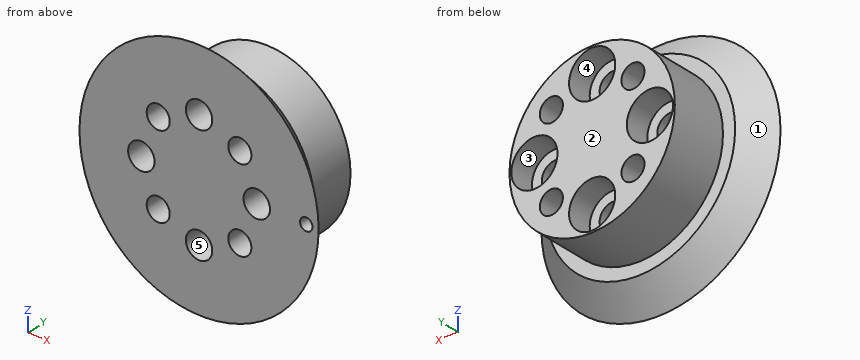
from build123d import *

# Parameters (mm, degrees)
SKETCH2_R                               = 1.4
CUT_EXTRUDE1_DEPTH                      = 23.814469093
CBORE_FOR_M5_HEX_HEAD_BOLT1_D           = 3.2
CBORE_FOR_M5_HEX_HEAD_BOLT1_CBORE_D     = 5.6
CBORE_FOR_M5_HEX_HEAD_BOLT1_CBORE_DEPTH = 3
SKETCH4_R                               = 0.75
CUT_EXTRUDE3_DEPTH                      = 23.814469093


with BuildPart() as part:
    # Sketch1 → Revolve1 (revolve)
    with BuildSketch(Plane.XY, mode=Mode.PRIVATE) as revolve1_sk:
        Polygon((14.5, 0), (11.5, 3), (10.025, 3), (10.025, 10), (0, 10), (0, 0), align=None)
    revolve(revolve1_sk.sketch.rotate(Axis((0, 10, 0), (0, -1, 0)), 180), axis=Axis((0, 10, 0), (0, -1, 0)))

    # Sketch2 → Cut-Extrude1 (cut, through all)
    with BuildSketch(Plane(origin=(0, 10, 0), x_dir=(1, 0, 0), z_dir=(0, 1, 0))):
        with Locations(Location((0, 7, 0), (0, 0, 180))):
            Circle(SKETCH2_R)
        with Locations(Location((4.949747468, 4.949747468, 0), (0, 0, 180))):
            Circle(SKETCH2_R)
        with Locations(Location((7, 0, 0), (0, 0, 180))):
            Circle(SKETCH2_R)
        with Locations(Location((4.949747468, -4.949747468, 0), (0, 0, 180))):
            Circle(SKETCH2_R)
        with Locations(Location((0, -7, 0), (0, 0, 180))):
            Circle(SKETCH2_R)
        with Locations(Location((-4.949747468, -4.949747468, 0), (0, 0, 180))):
            Circle(SKETCH2_R)
        with Locations(Location((-7, 0, 0), (0, 0, 180))):
            Circle(SKETCH2_R)
        with Locations(Location((-4.949747468, 4.949747468, 0), (0, 0, 180))):
            Circle(SKETCH2_R)
    extrude(amount=-CUT_EXTRUDE1_DEPTH, mode=Mode.SUBTRACT)

    # CBORE for M5 Hex Head Bolt1 (through all)
    with Locations(Plane(origin=(0, 10, -7), x_dir=(1, 0, 0), z_dir=(0, 1, 0))):
        with Locations((0, 0), (-7, -7), (0, -14), (7, -7)):
            CounterBoreHole(CBORE_FOR_M5_HEX_HEAD_BOLT1_D / 2, CBORE_FOR_M5_HEX_HEAD_BOLT1_CBORE_D / 2, CBORE_FOR_M5_HEX_HEAD_BOLT1_CBORE_DEPTH)

    # Sketch4 → Cut-Extrude3 (cut, through all)
    with BuildSketch(Plane(origin=(0, 0, 0), x_dir=(1, 0, 0), z_dir=(0, 1, 0))):
        with Locations(Location((13, 0, 0), (0, 0, 90.394644161))):
            Circle(SKETCH4_R)
    extrude(amount=CUT_EXTRUDE3_DEPTH, mode=Mode.SUBTRACT)


solid = part.part
Can you work these out from the model? Positions are in its coordinate system, mm. Face numbers are marked on the shaded views. A direction names the side the tool comes from. Coordinates: 2 decimals unless noted, no trailing zeros. Order: outer loops, then holes, each group sorted by start corner. A loop starts at its lowest first (then second) coordinate and runs counter-clockwise, first axis right, second up. Notation, with made-up numbers: (38, 29.25) - (71, 29.25) arc R25 cw to (71, 66.25) - close; hole circle Ø3 at (75.25, 88.5). An arc over 180 degrees is marked (long way). Answer as a JSON object with one key per item and string values. Group by question number.
Q1. Will these pins go through, and if not, where does the flat tip stop? P1, Ø2, axis at x = 4.95, z = 4.95, coming from the -Y side; P2, Ø6, axis at x = -11, y = 8.5, coming from the -Z side; P3, Ø5, axis at x = 0, z = -7, coming from the +Y side; P4, Ø1, axis at x = 9, y = 2.5, coming from the -Z side.
Q2. We'd pull the mould along Z, two halves only. Please class the marked faces 1, 2 and 3: +Z half, -Z half, draft (parallel to the pull), parting line (faces both ways), or undercut.
Q3. Imagine slicing it at A-A (z = 0). Please give me the cut outline in (x, y) (3 decimals), and give its area (3 significant figures).
Q4. I need wall thicknesses on line 1 (Z direction, x = 0, y = 9.05) (3 decimals); line 2 (X direction, y = 2.75, z = 0.25); line 3 (Z direction, x = -4, y = 1). Which ranges of each line are inside material? Lowest first, please. Write a range as from..to.
Q5. Imagine slicing it at B-B (x = 0). Please give me the cut outline in (y, z) (3 decimals), and give its area (3 significant figures).
Q6. On a 3-axis mill with a long thin cutter (end or side, diameter ignored), from which of +Z, -Z, +X, -X, +Y, -Y can I reach the whole of each face in a straight line? I mean the marked faces 4 and 5. Say none if no direction works.
Determined:
{
 "1": {"P1": "passes through", "P2": "stops at z = -6.04", "P3": "stops at y = 7", "P4": "stops at z = -8.84"},
 "2": {"face 1": "parting line", "face 2": "draft", "face 3": "undercut"},
 "3": {"outline": "(-14.5, 0) - (-8.6, 0) - (-8.6, 7) - (-9.8, 7) - (-9.8, 10) - (-10.025, 10) - (-10.025, 3) - (-11.5, 3) - close; (-5.4, 0) - (5.4, 0) - (5.4, 7) - (4.2, 7) - (4.2, 10) - (-4.2, 10) - (-4.2, 7) - (-5.4, 7) - close; (8.6, 0) - (12.25, 0) - (12.25, 2.25) - (11.5, 3) - (10.025, 3) - (10.025, 10) - (9.8, 10) - (9.8, 7) - (8.6, 7) - close; (13.75, 0) - (14.5, 0) - (13.75, 0.75) - close", "area": "138 mm2"},
 "4": {"line 1": "z = -10.025..-9.8, -4.2..4.2, 9.8..10.025", "line 2": "x = -11.75..-8.58, -5.42..5.42, 8.58..11.75", "line 3": "z = -12.89..-5.98, -3.92..3.92, 5.98..12.89"},
 "5": {"outline": "(0, -14.5) - (3, -11.5) - (3, -10.025) - (10, -10.025) - (10, -9.8) - (7, -9.8) - (7, -8.6) - (0, -8.6) - close; (0, -5.4) - (7, -5.4) - (7, -4.2) - (10, -4.2) - (10, 4.2) - (7, 4.2) - (7, 5.4) - (0, 5.4) - close; (0, 8.6) - (7, 8.6) - (7, 9.8) - (10, 9.8) - (10, 10.025) - (3, 10.025) - (3, 11.5) - (0, 14.5) - close", "area": "140 mm2"},
 "6": {"face 4": "+Y", "face 5": "+Y, -Y"}
}
